Geometry: final body of the model. Coordinates: model frame, mm. Face numbers are marked on the shaded views. A direction names the side the tool comes from. Give positions to 0.01 mm unless a question says otherwise; leave off trailing zeros. Loops run counter-clockwise (first coordinate to the right, second up) from the corner with the lowest first, then second, coordinate; pieces in that order, holes last. Notation, with made-up numbers: (88.25, 17.25) -> (122.25, 17.25) arc R21 ccw to (122.25, 44.25) -> close; hole circle Ø7 at (-17.75, -0.75). An arc over 180 degrees is marked (long way). One line per question, with ' | ' between items. Start each with the question number.
Item 1: Pin query (flat end, axial travel): P1, Ø1, axis at y = 5, z = 1.5, coming from the -X side; P2, Ø0.8, axis at x = 12, z = 1, coming from the +Y side. Return the tip coordinate at first contact, or that it passes through.
Item 2: Section A-A on y = 2.54. Return loops of the section in (x, z).
Item 3: Mould query, pull axis X, two halves, no side actions, for the marked faces 3, 4 and 5. Classes: released by +X, released by -X, zero draft, split by the parting line, or undercut.
Item 4: Set-up query: the marked faces 1 and 2. Return all of +Z, -Z, +X, -X, +Y, -Y with unobstructed straight access to the full face (end or side cutting, diameter ignored); none if empty.
Item 5: Section D-D on y = 6. Return loops of the section in (x, z), then the cut area to 3 significant figures.
Item 6: Section C-C on x = 12.7. Return loops of the section in (y, z).
Item 7: Section B-B on z = 0.85. Return loops of the section in (x, y).
Item 8: Material intervals for line 1 along Y through (x, z) = (12.7, 0.85); line 2 along Y through (x, z) = (14.75, 2.4); line 3 along X through (y, z) = (9, 1.4), sorted ascending. Write a range as [from, to].
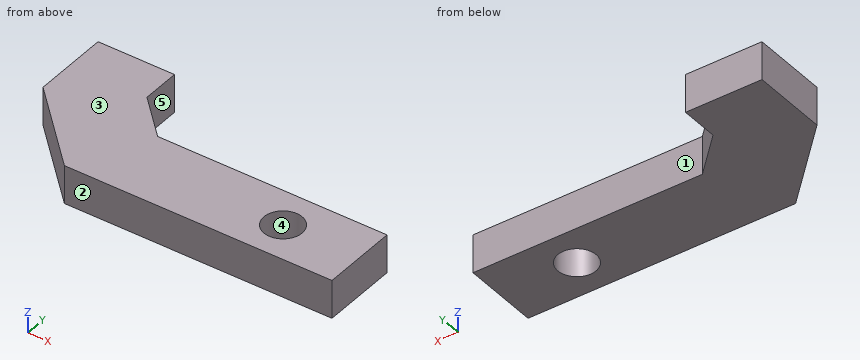
from build123d import *

# Parameters (mm, degrees)
BOSS_EXTRUDE1_DEPTH = 2.54
CUT_EXTRUDE1_REACH  = 4.54
SKETCH2_R           = 1.27


with BuildPart() as part:
    # Sketch1 → Boss-Extrude1 (new body)
    with BuildSketch(Plane.XY):
        Polygon((0, 0), (-5.08, 5.08), (-5.08, 10.16), (0, 10.16), (0, 7.62), (2.54, 5.08), (17.78, 5.08), (17.78, 0), align=None)
    extrude(amount=BOSS_EXTRUDE1_DEPTH)

    # Sketch2 → Cut-Extrude1 (cut, up to next)
    with BuildSketch(Plane.XY.offset(2.54), mode=Mode.PRIVATE) as cut_extrude1_sk1:
        with Locations((12.7, 2.54)):
            Circle(SKETCH2_R)
    cut_extrude1_tool1 = extrude(cut_extrude1_sk1.sketch, amount=-CUT_EXTRUDE1_REACH, mode=Mode.PRIVATE) & part.part
    add(cut_extrude1_tool1.solids().sort_by_distance((12.7, 2.54, 2.54))[0], mode=Mode.SUBTRACT)


solid = part.part
Result sheet:
1) P1: stops at x = -5.08 | P2: stops at y = 5.08
2) outline: (-2.54, 0) -> (11.43, 0) -> (11.43, 2.54) -> (-2.54, 2.54) -> close; (13.97, 0) -> (17.78, 0) -> (17.78, 2.54) -> (13.97, 2.54) -> close
3) face 3: zero draft | face 4: undercut | face 5: released by +X
4) face 1: +Z, -Z, +X, +Y | face 2: +Z, -Z, +X, -X, -Y
5) outline: (-5.08, 0) -> (1.62, 0) -> (1.62, 2.54) -> (-5.08, 2.54) -> close | area: 17.0 mm²
6) outline: (0, 0) -> (1.27, 0) -> (1.27, 2.54) -> (0, 2.54) -> close; (3.81, 0) -> (5.08, 0) -> (5.08, 2.54) -> (3.81, 2.54) -> close
7) outline: (-5.08, 5.08) -> (0, 0) -> (17.78, 0) -> (17.78, 5.08) -> (2.54, 5.08) -> (0, 7.62) -> (0, 10.16) -> (-5.08, 10.16) -> close; hole circle Ø2.54 at (12.7, 2.54)
8) line 1: y = [0, 1.27], [3.81, 5.08] | line 2: y = [0, 5.08] | line 3: x = [-5.08, 0]
